```python
from build123d import *

# Parameters (mm, degrees)
SKETCH_W        = 28.817356
SKETCH_H        = 24.401199
PAD_DEPTH       = 10
SKETCH001_R     = 3.449545
POCKET_DEPTH    = 10.001
SKETCH002_R     = 2.5
POCKET001_DEPTH = 5


with BuildPart() as part:
    # Sketch → Pad (new body)
    with BuildSketch(Plane.XY):
        with Locations((14.408678, 12.200599)):
            Rectangle(SKETCH_W, SKETCH_H)
    extrude(amount=PAD_DEPTH)

    # Sketch001 → Pocket (cut, through all)
    with BuildSketch(Plane.XY):
        with Locations((5.970357, 10.013991)):
            Circle(SKETCH001_R)
    extrude(amount=POCKET_DEPTH, mode=Mode.SUBTRACT)

    # Sketch002 (on Face5 of Pocket) → Pocket001 (cut)
    with BuildSketch(Plane.XY.offset(10)):
        with Locations((22.960093, 5.495847)):
            Circle(SKETCH002_R)
        with Locations((22.960093, 20.067438)):
            Circle(SKETCH002_R)
    extrude(amount=-POCKET001_DEPTH, mode=Mode.SUBTRACT)


solid = part.part
```
Geometry: final body of the model. Coordinates: model frame, mm. A direction names the side the tool comes from. Give positions to 0.01 mm unless a question says otherwise; leave off trailing zeros. Write each loop counter-clockwise with the first axis right and the second up, starting at its lowest first coordinate (ties: lowest second). Pieces come first, ordered by that corner, then holes.
1. Reachability of faces 5 (the cylindrical face through (7.825, 12.923, 4.93)), 6 (the cylindrical face through (22.418, 17.627, 7.535)) from +Z, -Z, +X, -X, +Y, -Y: full face, straight path, thin tool, end or side. Return the list, or none.
2. Line query: probe 1 along X at (y, z) = (7, 8.5); probe 2 along Y at (x, z) = (22.25, 8); probe 3 along Y at (x, z) = (21.5, 8.75). Output: solid intervals per line, ascending.
3. Section query D-D, the plane y = 19.5. Return loops of the section in (x, z), then the cut area to 3 significant figures.
4. Section query B-B, the plane y = 12. Return loops of the section in (x, z), then the cut area to 3 significant figures.
5. Section query C-C, the plane z = 8.5. Return loops of the section in (x, y), then the cut area to 3 significant figures.
6. Draft query along Y for faces 1 (the flat face through (23, 6, 5)), 2 (the flat face through (14, 12, 10)), 3 (the flat face through (14, 24.401, 5)), 4 (the flat face through (14, 0, 5)). Return one class per face: released by +Y, released by -Y, zero draft, split by the parting line, or undercut.
7. Section query A-A, the plane x = 7.75. Return loops of the section in (y, z).
8. Pin query (flat end, axial travel): P1, Ø6, axis at x = 5.97, y = 10.01, coming from the +Z side; P2, Ø3, axis at x = 22.96, y = 5.5, coming from the +Z side. Return the tip coordinate at first contact, or that it passes through.
Computed:
1. face 5: +Z, -Z
1. face 6: +Z
2. probe 1: x = 0 to 4.29, 7.65 to 20.96, 24.96 to 28.82
2. probe 2: y = 0 to 3.1, 7.89 to 17.67, 22.46 to 24.4
2. probe 3: y = 0 to 3.47, 7.53 to 18.04, 22.1 to 24.4
3. outline: (0, 0) - (28.82, 0) - (28.82, 10) - (25.39, 10) - (25.39, 5) - (20.53, 5) - (20.53, 10) - (0, 10) - close
3. area: 264 mm2
4. outline: (0, 0) - (3.15, 0) - (3.15, 10) - (0, 10) - close; (8.79, 0) - (28.82, 0) - (28.82, 10) - (8.79, 10) - close
4. area: 232 mm2
5. outline: (0, 0) - (28.82, 0) - (28.82, 24.4) - (0, 24.4) - close; hole circle Ø6.9 at (5.97, 10.01); hole circle Ø5 at (22.96, 5.5); hole circle Ø5 at (22.96, 20.07)
5. area: 627 mm2
6. face 1: undercut
6. face 2: zero draft
6. face 3: released by +Y
6. face 4: released by -Y
7. outline: (0, 0) - (7.06, 0) - (7.06, 10) - (0, 10) - close; (12.97, 0) - (24.4, 0) - (24.4, 10) - (12.97, 10) - close
8. P1: passes through
8. P2: stops at z = 5
